Model file for the job. Use its own axes, mm. Face numbers are marked on the shaded views. A direction names the side the tool comes from. Give positions to 0.01 mm unless a question says otherwise; leave off trailing zeros. Loops run counter-clockwise (first coordinate to the right, second up) from the corner with the lowest first, then second, coordinate; pieces in that order, holes last. Notation, with made-up numbers: M 46.25,80 L 78.25,80 A12 ccw 78.25,92 Z; hole C -13.75,-39 d4. An arc over 180 degrees is marked long. Use CSV: the item, a comma, the result in double quotes. Start each with the question number.
(1) Two-plate mould, pull along Z, no slides. Class the marked faces 1, 2 and 3: pulls with the +Z half, pulls with the -Z half, needs draft (parallel to the pull), parting line crosses it, or undercut.
(2) Slice it at C-C on z = 6.5. List the corners of the cut face in (x, y), and give its area (3 significant figures).
(3) Tool access for the marked faces 4 and 5: list every direction of +Z, -Z, +X, -X, +Y, -Y with a clear straight run to the whole face (end or side of a thin tool).
(4) Slice it at B-B on z = 4.15. List the corners of the cut face in (x, y).
(5) Flat gauge pin, fed straight in: P1, Ø4.5, axis at x = -7.6, z = 4.15, coming from the +Y side. Where does the tip first touch, or does it go through?
(6) Slice it at D-D on y = 10.25. List the corners of the cut face in (x, z).
(7) Wall check: line 1 along X through (y, z) = (9, 4.25); line 2 along X through (y, z) = (12, 2.75); line 3 along X through (y, z) = (3, 5.5). Give the ranges that are in metal, low to high. Write a range as from..to.
(8) Slice it at A-A on x = 7.6. List the corners of the cut face in (y, z), and give its area (3 significant figures).
```python
from build123d import *

# Parameters (mm, degrees)
SKETCH1_W           = 20.2
SKETCH1_H           = 13.3
SKETCH1_R           = 1.75
BOSS_EXTRUDE1_DEPTH = 11.8
BOSS_EXTRUDE2_DEPTH = 12.8


with BuildPart() as part:
    # Sketch1 → Boss-Extrude1 (new body)
    # profile 1 of 2: a face of its own
    with BuildSketch(Plane(origin=(0, 0, 0), x_dir=(1, 0, 0), z_dir=(0, 1, 0))):
        Rectangle(SKETCH1_W, SKETCH1_H)
        with Locations(Location((-7.6, -4.15, 0), (0, 0, 270))):
            Circle(SKETCH1_R, mode=Mode.SUBTRACT)
        with Locations(Location((7.6, -4.15, 0), (0, 0, 270))):
            Circle(SKETCH1_R, mode=Mode.SUBTRACT)
    # profile 2 of 2: a face of its own
    with BuildSketch(Plane(origin=(0, 0, 0), x_dir=(1, 0, 0), z_dir=(0, 1, 0))):
        Polygon((11.1, -7.65), (11.1, 6.65), (10.1, 6.65), (10.1, -6.65), (-10.1, -6.65), (-10.1, 6.65), (-11.1, 6.65), (-11.1, -7.65), align=None)
    extrude(amount=BOSS_EXTRUDE1_DEPTH)

    # Sketch1_3 → Boss-Extrude2 (add)
    with BuildSketch(Plane(origin=(0, 0, 0), x_dir=(1, 0, 0), z_dir=(0, 1, 0))):
        Polygon((12.1, -8.65), (12.1, 6.65), (11.1, 6.65), (11.1, -7.65), (-11.1, -7.65), (-11.1, 6.65), (-12.1, 6.65), (-12.1, -8.65), align=None)
    extrude(amount=BOSS_EXTRUDE2_DEPTH)


solid = part.part
```
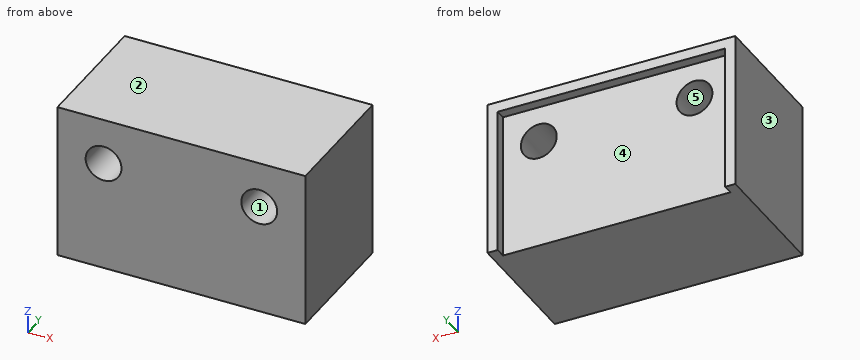
Reply:
1,face 1,"undercut"
1,face 2,"pulls with the +Z half"
1,face 3,"needs draft"
2,outline,"M -12.1,0 L 12.1,0 L 12.1,12.8 L 11.1,12.8 L 11.1,11.8 L -11.1,11.8 L -11.1,12.8 L -12.1,12.8 Z"
2,area,"288 mm^2"
3,face 4,"-Z, +Y"
3,face 5,"+Y, -Y"
4,outline,"M -12.1,0 L -9.35,0 L -9.35,11.8 L -11.1,11.8 L -11.1,12.8 L -12.1,12.8 Z; M -5.85,0 L 5.85,0 L 5.85,11.8 L -5.85,11.8 Z; M 9.35,0 L 12.1,0 L 12.1,12.8 L 11.1,12.8 L 11.1,11.8 L 9.35,11.8 Z"
5,P1,"stops at y = 11.8"
6,outline,"M -12.1,-6.65 L 12.1,-6.65 L 12.1,8.65 L -12.1,8.65 Z; hole C -7.6,4.15 d3.5; hole C 7.6,4.15 d3.5"
7,line 1,"x = -12.1..-9.35, -5.85..5.85, 9.35..12.1"
7,line 2,"x = -12.1..-11.1, 11.1..12.1"
7,line 3,"x = -12.1..-8.71, -6.49..6.49, 8.71..12.1"
8,outline,"M 0,-6.65 L 11.8,-6.65 L 11.8,2.4 L 0,2.4 Z; M 0,5.9 L 11.8,5.9 L 11.8,7.65 L 12.8,7.65 L 12.8,8.65 L 0,8.65 Z"
8,area,"140 mm^2"
